```python
from build123d import *

# Parameters (mm, degrees)
SKETCH2_R           = 22.225
SKETCH2_R_2         = 3.175
BOSS_EXTRUDE1_DEPTH = 6.35
SKETCH3_R           = 2.0828
CUT_EXTRUDE1_DEPTH  = 6.35


with BuildPart() as part:
    # Sketch2 → Boss-Extrude1 (new body)
    with BuildSketch(Plane(origin=(0, 0, 0), x_dir=(1, 0, 0), z_dir=(0, 1, 0))):
        with BuildLine():
            Line((-34.29, -44.45), (34.29, -44.45))
            ThreePointArc((34.29, -44.45), (41.474204897, -41.474204897), (44.45, -34.29))
            Line((44.45, -34.29), (44.45, 34.29))
            ThreePointArc((44.45, 34.29), (41.474204897, 41.474204897), (34.29, 44.45))
            Line((34.29, 44.45), (-34.29, 44.45))
            ThreePointArc((-34.29, 44.45), (-41.474204897, 41.474204897), (-44.45, 34.29))
            Line((-44.45, 34.29), (-44.45, -34.29))
            ThreePointArc((-44.45, -34.29), (-41.474204897, -41.474204897), (-34.29, -44.45))
        make_face()
        with Locations(Location((0, 0, 0), (0, 0, 270))):
            Circle(SKETCH2_R, mode=Mode.SUBTRACT)
        with Locations(Location((-34.925, 34.925, 0), (0, 0, 270))):
            Circle(SKETCH2_R_2, mode=Mode.SUBTRACT)
        with Locations(Location((34.925, 34.925, 0), (0, 0, 90))):
            Circle(SKETCH2_R_2, mode=Mode.SUBTRACT)
        with Locations(Location((34.925, -34.925, 0), (0, 0, 270))):
            Circle(SKETCH2_R_2, mode=Mode.SUBTRACT)
        with Locations(Location((-34.925, -34.925, 0), (0, 0, 90))):
            Circle(SKETCH2_R_2, mode=Mode.SUBTRACT)
    extrude(amount=BOSS_EXTRUDE1_DEPTH)

    # Sketch3 → Cut-Extrude1 (cut)
    with BuildSketch(Plane(origin=(0, 6.35, 0), x_dir=(1, 0, 0), z_dir=(0, 1, 0))):
        with Locations(Location((26.67, 0, 0), (0, 0, 270))):
            Circle(SKETCH3_R)
        with Locations(Location((18.858537854, -18.858537854, 0), (0, 0, 270))):
            Circle(SKETCH3_R)
        with Locations(Location((0, -26.67, 0), (0, 0, 270))):
            Circle(SKETCH3_R)
        with Locations(Location((-18.858537854, -18.858537854, 0), (0, 0, 270))):
            Circle(SKETCH3_R)
        with Locations(Location((-26.67, 0, 0), (0, 0, 270))):
            Circle(SKETCH3_R)
        with Locations(Location((-18.858537854, 18.858537854, 0), (0, 0, 270))):
            Circle(SKETCH3_R)
        with Locations(Location((0, 26.67, 0), (0, 0, 270))):
            Circle(SKETCH3_R)
        with Locations(Location((18.858537854, 18.858537854, 0), (0, 0, 270))):
            Circle(SKETCH3_R)
    extrude(amount=-CUT_EXTRUDE1_DEPTH, mode=Mode.SUBTRACT)


solid = part.part
```
Design review of the part built by this model. Coordinates are the model's own, in mm. Give positions to 0.01 mm unless a question says otherwise; leave off trailing zeros. Order: outer loops, then holes, each group sorted by start corner. A loop starts at its lowest first (then second) coordinate and runs counter-clockwise, first axis right, second up. Notation, with made-up numbers: M 58.5,-32.75 L 67.5,-32.75 A16 cw 67.5,-24.75 Z; hole C 24.25,36.5 d4. An arc over 180 degrees is marked long. One line per question, with ' | ' between items. Start each with the question number.
Q1. We need section A-A (x = 0). Write out the cut boundary in (y, z) (3 decimals), plus the area to 3 significant figures.
Q2. The part is to be moulded in two halves that separate along Z. For faces 1 (the face through (0, 3, -44.45)), 2 (the face through (-11, 6.35, -20)), 3 (the face through (-37.602, 3.131, 33.218)), say which applies: +Z half, -Z half, draft (parallel to the pull), parting line (faces both ways), or undercut.
Q3. We need section B-B (z = 0). Write out the cut boundary in (x, y) (3 decimals), plus the area to 3 significant figures.
Q4. For pin 1 Ø3.5 at (x, z) = (0, 26.67) entering from +Y, flat-tipped, find the tip position at first contact; note if it passes through.
Q5. We need section C-C (x = 26.67). Write out the cut boundary in (y, z), plus the area to 3 significant figures.
Q6. We need section D-D (z = -26.67). Write out the cut boundary in (x, y).
Q7. For L1, parallel to Z at x = 35.5, y = 3.25; L2, parallel to X at y = 4.5, z = 32; L3, parallel to X at y = 3.25, z = -20, list the stretches that pass through material, from the lowest coordinate up. Write a range as [from, to].
Returned:
1) outline: M 0,-44.45 L 6.35,-44.45 L 6.35,-28.753 L 0,-28.753 Z; M 0,-24.587 L 6.35,-24.587 L 6.35,-22.225 L 0,-22.225 Z; M 0,22.225 L 6.35,22.225 L 6.35,24.587 L 0,24.587 Z; M 0,28.753 L 6.35,28.753 L 6.35,44.45 L 0,44.45 Z | area: 229 mm2
2) face 1: -Z half | face 2: draft | face 3: undercut
3) outline: M -44.45,0 L -28.753,0 L -28.753,6.35 L -44.45,6.35 Z; M -24.587,0 L -22.225,0 L -22.225,6.35 L -24.587,6.35 Z; M 22.225,0 L 24.587,0 L 24.587,6.35 L 22.225,6.35 Z; M 28.753,0 L 44.45,0 L 44.45,6.35 L 28.753,6.35 Z | area: 229 mm2
4) pin 1: through
5) outline: M 0,-44.45 L 6.35,-44.45 L 6.35,-2.08 L 0,-2.08 Z; M 0,2.08 L 6.35,2.08 L 6.35,44.45 L 0,44.45 Z | area: 538 mm2
6) outline: M -44.45,0 L -2.08,0 L -2.08,6.35 L -44.45,6.35 Z; M 2.08,0 L 44.45,0 L 44.45,6.35 L 2.08,6.35 Z
7) L1: [-44.38, -38.05], [-31.8, 31.8], [38.05, 44.38] | L2: [-44.45, -36.16], [-33.69, 33.69], [36.16, 44.45] | L3: [-44.45, -20.6], [-17.12, -9.69], [9.69, 17.12], [20.6, 44.45]
